from build123d import *

# Parameters (mm, degrees)
SKETCH1_W           = 29
SKETCH1_H           = 47
BOSS_EXTRUDE1_DEPTH = 26
SHELL1_T            = -3
SKETCH2_W           = 10
SKETCH2_H           = 8.23076923
CUT_EXTRUDE1_DEPTH  = 26
SKETCH3_W           = 29
SKETCH3_H           = 26
BOSS_EXTRUDE2_DEPTH = 16
SKETCH4_R           = 2.5
CUT_EXTRUDE2_DEPTH  = 62.040969848
SKETCH5_W           = 29
SKETCH5_H           = 50
SKETCH5_R           = 2.38125
BOSS_EXTRUDE3_DEPTH = 4


with BuildPart() as part:
    # Sketch1 → Boss-Extrude1 (new body)
    with BuildSketch(Plane.XY):
        with Locations((14.5, 23.5)):
            Rectangle(SKETCH1_W, SKETCH1_H)
    extrude(amount=BOSS_EXTRUDE1_DEPTH)

    # Shell1
    shell1_openings = [part.faces().sort_by_distance(p)[0] for p in [
        (0, 23.5, 13),
    ]]
    offset(amount=SHELL1_T, openings=shell1_openings, kind=Kind.INTERSECTION)

    # Sketch2 → Cut-Extrude1 (cut)
    with BuildSketch(Plane.ZY):
        with Locations((13, 44)):
            Rectangle(SKETCH2_W, SKETCH2_H)
    extrude(amount=-CUT_EXTRUDE1_DEPTH, mode=Mode.SUBTRACT)

    # Sketch3 → Boss-Extrude2 (add)
    with BuildSketch(Plane.XZ):
        with Locations((14.5, 13)):
            Rectangle(SKETCH3_W, SKETCH3_H)
    extrude(amount=BOSS_EXTRUDE2_DEPTH)

    # Sketch4 → Cut-Extrude2 (cut, through all)
    with BuildSketch(Plane.ZY):
        with Locations(Location((8, -2, 0), (0, 0, 270))):
            Circle(SKETCH4_R)
        with Locations(Location((18, -2, 0), (0, 0, 270))):
            Circle(SKETCH4_R)
    extrude(amount=-CUT_EXTRUDE2_DEPTH, mode=Mode.SUBTRACT)

    # Sketch5 → Boss-Extrude3 (add)
    with BuildSketch(Plane.XZ.offset(16)):
        with Locations((14.5, 13)):
            Rectangle(SKETCH5_W, SKETCH5_H)
        with Locations(Location((14.5, 31, 0), (0, 0, 270))):
            Circle(SKETCH5_R, mode=Mode.SUBTRACT)
        with Locations(Location((14.5, -5, 0), (0, 0, 270))):
            Circle(SKETCH5_R, mode=Mode.SUBTRACT)
    extrude(amount=BOSS_EXTRUDE3_DEPTH)


solid = part.part
Design review of the part built by this model. Coordinates are the model's own, in mm. A direction names the side the tool comes from. Round coordinates to 2 decimals unless told otherwise and drop trailing zeros. Write each loop counter-clockwise with the first axis right and the second up, starting at its lowest first coordinate (ties: lowest second). Pieces come first, ordered by that corner, then holes. Notation, with made-up numbers: M 61.5,78.25 L 80.5,78.25 A27 ccw 80.5,107.25 Z; hole C 5.5,-29.75 d5. An arc over 180 degrees is marked long. One line per item, written item: value. Start each with the question number.
1. Take a section at A-A on x = 14.5. State the section outline as (y, z) points, then the cut area to 3 significant figures.
2. For faces 1 (the face through (14, 16, 26)), 2 (the face through (13, 3, 13)), 3 (the face through (13, 45, 18)), list the 3-axis set-ups (+Z, -Z, +X, -X, +Y, -Y) from which the entire face can be reached by the end or side of a thin tool; tool diameter is ignored.
3. Take a section at C-C on z = -5. State the section outline as (x, y) points.
4. Take a section at D-D on x = 24. State the section outline as (y, z) points.
5. Clearance check with flat-ended pins moving along their axes: P1, Ø5, axis at x = 5.5, y = -11, coming from the -Z side; P2, Ø0.9, axis at x = 17, y = 45.5, coming from the +Z side; P3, Ø3, axis at y = -2, z = 8, coming from the -X side; P4, Ø6, axis at x = 9, z = -8, coming from the +Y side. State where each tip first meets the part, or that it passes through.
6. To check wall thickness, follow probe 1 along Z at (x, y) = (13.5, -2); probe 2 along Z at (x, y) = (5.25, 14.5); probe 3 along Y at (x, z) = (8, 19). State the ranges of each line that lie inside material, in increasing order. Write a range as from..to.
7. Draft analysis for pull direction X (two halves, no side actions). For faces 4 (the face through (13, 44, 20)), 5 (the face through (0, 1, 15)), 6 (the face through (14.6, -17.97, 33.38)), state which applies: pulls with the +X half, pulls with the -X half, needs draft (parallel to the pull), parting line crosses it, or undercut.
8. Take a section at B-B on y = -2. State the section outline as (x, z) points.
Computed:
1. outline: M -20,-12 L -16,-12 L -16,-7.38 L -20,-7.38 Z; M -20,-2.62 L -16,-2.62 L -16,0 L 47,0 L 47,8 L 44,8 L 44,3 L 3,3 L 3,23 L 44,23 L 44,18 L 47,18 L 47,26 L -16,26 L -16,28.62 L -20,28.62 Z; M -20,33.38 L -16,33.38 L -16,38 L -20,38 Z; hole C -2,8 d5; hole C -2,18 d5
1. area: 911 mm²
2. face 1: +Z, +X, -X, +Y
2. face 2: -X
2. face 3: -X, +Y
3. outline: M 0,-20 L 12.12,-20 L 12.12,-16 L 0,-16 Z; M 16.88,-20 L 29,-20 L 29,-16 L 16.88,-16 Z
4. outline: M -20,-12 L -16,-12 L -16,0 L 47,0 L 47,8 L 44,8 L 44,3 L 3,3 L 3,23 L 44,23 L 44,18 L 47,18 L 47,26 L -16,26 L -16,38 L -20,38 Z; hole C -2,8 d5; hole C -2,18 d5
5. P1: stops at z = 0
5. P2: stops at z = 26
5. P3: passes through
5. P4: stops at y = -16
6. probe 1: z = 0..5.5, 10.5..15.5, 20.5..26
6. probe 2: z = 0..3, 23..26
6. probe 3: y = -20..-4.29, 0.29..3, 44..47
7. face 4: needs draft
7. face 5: pulls with the -X half
7. face 6: undercut
8. outline: M 0,0 L 29,0 L 29,5.5 L 0,5.5 Z; M 0,10.5 L 29,10.5 L 29,15.5 L 0,15.5 Z; M 0,20.5 L 29,20.5 L 29,26 L 0,26 Z
